Source: CAD feature listing. Evaluate the final solid. Frame: model axes, mm. A direction names the side the tool comes from. Give positions to 0.01 mm unless a question says otherwise; leave off trailing zeros. Order: outer loops, then holes, each group sorted by start corner. A loop starts at its lowest first (then second) coordinate and runs counter-clockwise, first axis right, second up. Notation, with made-up numbers: M -27.75,19.25 L -7.75,19.25 A11 ccw -7.75,31.25 Z; hole C 53.25,69.5 d10. An arc over 180 degrees is marked long. Answer in a Markdown table with one row per item. Add a question column.
(1) Section query A-A, the plane y = 10. Return loops of the section in (x, z).
(2) Section query C-C, the plane z = 3.25. Return loops of the section in (x, y).
(3) Set-up query: faces 5 (the face through (75, 20, 5)), 6 (the face through (-2.722, 0.378, 4.93)). Return all of +Z, -Z, +X, -X, +Y, -Y with unobstructed straight access to the full face (end or side cutting, diameter ignored); none if empty.
(4) Mould query, pull axis Y, two halves, no side actions, for faces 1 (the face through (162, 10, 5)), 2 (the face through (-22.6, 27.3, 4.9)), 3 (the face through (-0.54, 7.56, 4.93)), 4 (the face through (-16.531, 9.887, 4.93)). Classes: pulls with the +Y half, pulls with the -Y half, needs draft (parallel to the pull), parting line crosses it, or undercut.
(5) Material intervals for line 1 along Y through (x, z) = (0, 5.25); line 2 along X through (y, z) = (9.5, 4.75); line 3 along X through (y, z) = (10.5, 7.5), sorted ascending.
(6) Pin query (flat end, axial travel): P1, Ø3, axis at x = 54.5, z = 3.5, coming from the +Y side; P2, Ø1.5, axis at y = 14, z = 9, coming from the -X side. Return the tip coordinate at first contact, or that it passes through.
(7) Section query B-B, the plane x = 104.5. Return loops of the section in (y, z).
from build123d import *

# Parameters (mm, degrees)
ESQUISSE1_R        = 2.5
ESQUISSE1_R_2      = 1.5
BOSS_EXTRU_1_DEPTH = 10


with BuildPart() as part:
    # Esquisse1 → Boss.-Extru.1 (new body)
    with BuildSketch(Plane.XY):
        with BuildLine():
            Line((-5.305683683, 1.523578547), (-28.075920727, 18.488824386))
            ThreePointArc((-28.075920727, 18.488824386), (-30.036088987, 21.775525063), (-29.098088919, 25.485621667))
            Line((-29.098088919, 25.485621667), (-24.762545303, 31.304656462))
            ThreePointArc((-24.762545303, 31.304656462), (-21.496491478, 33.261764377), (-17.799326826, 32.351625643))
            Line((-17.799326826, 32.351625643), (-0.876599726, 19.961504551))
            ThreePointArc((-0.876599726, 19.961504551), (-0.438722287, 19.990371502), (0, 20))
            Line((0, 20), (152, 20))
            ThreePointArc((152, 20), (162, 10), (152, 0))
            Line((152, 0), (0, 0))
            ThreePointArc((0, 0), (-2.760053031, 0.388438875), (-5.305683683, 1.523578547))
        make_face()
        with Locations((0, 10)):
            Circle(ESQUISSE1_R, mode=Mode.SUBTRACT)
        with Locations((152, 10)):
            Circle(ESQUISSE1_R, mode=Mode.SUBTRACT)
        with Locations((-23.409755192, 26.035431675)):
            Circle(ESQUISSE1_R_2, mode=Mode.SUBTRACT)
    extrude(amount=BOSS_EXTRU_1_DEPTH)


solid = part.part
Values follow:
| question | item | result |
|---|---|---|
| 1 | outline | M -16.68,0 L -2.5,0 L -2.5,10 L -16.68,10 Z; M 2.5,0 L 149.5,0 L 149.5,10 L 2.5,10 Z; M 154.5,0 L 162,0 L 162,10 L 154.5,10 Z |
| 2 | outline | M -29.1,25.49 A5 ccw -28.08,18.49 L -5.31,1.52 A10 ccw 0,0 L 152,0 A10 ccw 152,20 L 0,20 A10 ccw -0.88,19.96 L -17.8,32.35 A5 ccw -24.76,31.3 Z; hole C -23.41,26.04 d3; hole C 0,10 d5; hole C 152,10 d5 |
| 3 | face 5 | +Z, -Z, +X, +Y |
| 3 | face 6 | +Z, -Z, -X, -Y |
| 4 | face 1 | parting line crosses it |
| 4 | face 2 | undercut |
| 4 | face 3 | undercut |
| 4 | face 4 | pulls with the -Y half |
| 5 | line 1 | y = 0 to 7.5, 12.5 to 20 |
| 5 | line 2 | x = -16.01 to -2.45, 2.45 to 149.55, 154.45 to 161.99 |
| 5 | line 3 | x = -17.35 to -2.45, 2.45 to 149.55, 154.45 to 161.99 |
| 6 | P1 | stops at y = 20 |
| 6 | P2 | stops at x = -23.06 |
| 7 | outline | M 0,0 L 20,0 L 20,10 L 0,10 Z |
